```python
from build123d import *

# Parameters (mm, degrees)
F1_DEPTH = 7.62
F0_W     = 4.7625
F0_H     = 7.9375
F2_DEPTH = 4.7752
F3_DEPTH = 3.175


with BuildPart() as f1:
    # F0 (on Top) → F1 (new body)
    with BuildSketch(Plane.XY):
        Polygon((0, -18.387259), (-4.7625, -18.387259), (-7.9375, -18.387259), (-7.9375, -19.974759), (3.175, -19.974759), (3.175, -18.387259), align=None)
    extrude(amount=F1_DEPTH)

    # F0 (on Top) → F2 (join)
    with BuildSketch(Plane.XY):
        with Locations((-2.38125, -14.418509)):
            Rectangle(F0_W, F0_H)
        with BuildLine():
            Line((-1.394904, -7.082163), (-4.7625, -10.449759))
            Line((-4.7625, -10.449759), (0, -10.449759))
            ThreePointArc((0, -10.449759), (-0.362524, -8.627229), (-1.394904, -7.082163))
        make_face()
        Polygon((-10.146717, -5.065542), (-4.7625, -10.449759), (-1.394904, -7.082163), (-6.779121, -1.697946), align=None)
    extrude(amount=F2_DEPTH)


with BuildPart() as f3:
    # F0 (on Top) → F3 (new body)
    with BuildSketch(Plane.XY):
        Polygon((30.061543, 3.299114), (11.011543, 3.299114), (11.011543, -22.100886), (49.111543, -22.100886), (49.111543, 3.299114), align=None)
        Polygon((27.521543, -6.860886), (30.061543, -6.860886), (32.601543, -6.860886), (32.601543, -11.940886), (27.521543, -11.940886), align=None, mode=Mode.SUBTRACT)
    extrude(amount=F3_DEPTH)


solid = f1.part
```
Could you check a few things on this model? Use its own coordinates, in mm. A direction names the side the tool comes from. Coordinates: 2 decimals unless noted, no trailing zeros. Loops run counter-clockwise (first coordinate to the right, second up) from the corner with the lowest first, then second, coordinate; pieces in that order, holes last. Notation, with made-up numbers: M 72.5,12.5 L 79.5,12.5 A8 ccw 79.5,18.5 Z; hole C 59.25,-25 d4. An arc over 180 degrees is marked long. Put each result on its own line as item: value. Start each with the question number.
(1) I need wall thicknesses on line 1 (Y direction, x = 2, z = 4.25); line 2 (X direction, y = -11.25, z = 2.5); line 3 (Z direction, x = -2.25, y = -17.5). Which ranges of each line are inside material? Lowest first, please. Write a range as from..to.
(2) Suppose I cut it at B-B on z = 2.75. Please give me the cut outline in (x, y) (1 decimal).
(3) Thinking about a two-plate mould opening in Y: for faces 1 (the face through (-2, -19.975, 4)), 2 (the face through (-0.353, -8.651, 2.354)), 3 (the face through (-2, -18.387, 5)), 4 (the face through (-2, -19, 7.62)), which applies, pulls with the +Y half, pulls with the -Y half, needs draft (parallel to the pull), parting line crosses it, or undercut?
(4) Suppose I cut it at C-C on y = -13.5. Please give me the cut outline in (x, z).
(5) Will these pins go through, and if not, where does the flat tip stop? P1, Ø5, axis at x = -6, y = -9, coming from the +Z side; P2, Ø1.4, axis at y = -15.5, z = 3, coming from the +X side; P3, Ø1.3, axis at y = -19.5, z = 5, coming from the -X side.
(6) Suppose I cut it at A-A on x = -7.5. Please give me the cut outline in (y, z).
(7) For faces 5 (the face through (0, -14, 2)), 6 (the face through (-7.938, -19, 4)), 7 (the face through (-4, -10, 4.775)), 8 (the face through (-7.49, -7.72, 2.35)), which set-ups out of +Z, -Z, +X, -X, +Y, -Y let a thin tool reach every point of the face, with its end or its side?
(8) Suppose I cut it at D-D on x = 0.25. Please give me the cut outline in (y, z).
Solutions:
1. line 1: y = -19.97..-18.39
1. line 2: x = -4.76..0
1. line 3: z = 0..4.78
2. outline: M -10.1,-5.1 L -4.8,-10.4 L -4.8,-18.4 L -7.9,-18.4 L -7.9,-20 L 3.2,-20 L 3.2,-18.4 L 0,-18.4 L 0,-10.4 A4.8 ccw -1.4,-7.1 L -6.8,-1.7 Z
3. face 1: pulls with the -Y half
3. face 2: pulls with the +Y half
3. face 3: undercut
3. face 4: needs draft
4. outline: M -4.76,0 L 0,0 L 0,4.78 L -4.76,4.78 Z
5. P1: stops at z = 4.78
5. P2: stops at x = 0
5. P3: stops at x = -7.94
6. outline: M -19.97,0 L -18.39,0 L -18.39,7.62 L -19.97,7.62 Z; M -7.71,0 L -2.42,0 L -2.42,4.78 L -7.71,4.78 Z
7. face 5: +Z, -Z, +X, +Y
7. face 6: +Z, -Z, -X, -Y
7. face 7: +Z, +X, -X, +Y
7. face 8: +Z, -Z, -X
8. outline: M -19.97,0 L -18.39,0 L -18.39,7.62 L -19.97,7.62 Z
